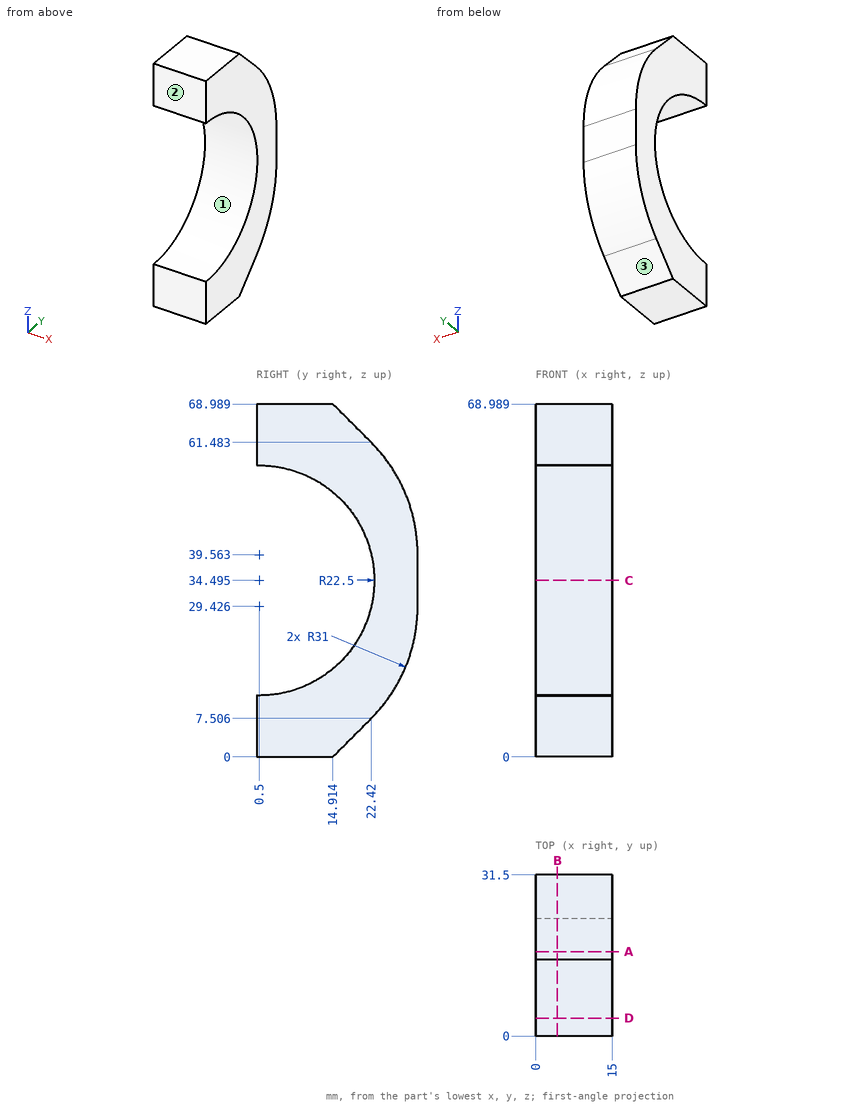
The drawing under review shows one solid part. Ordinate dimensions are in mm from its lowest x, y, z. Round coordinates to 2 decimals unless told otherwise and drop trailing zeros. Loops run counter-clockwise (first coordinate to the right, second up) from the corner with the lowest first, then second, coordinate; pieces in that order, holes last. Notation, with made-up numbers: (-21, 3) - (21, 3) arc R10 cw to (21, 21) - close; hole circle Ø6 at (-26, 18.5). An arc over 180 degrees is marked (long way). Use a Markdown table: item, result. Add a question column.
Q1. Add section B-B (x = 4.25). State the section outline as (y, z) points (1 decimal).
Q2. Add section C-C (z = 34.5). State the section outline as (x, y) points.
Q3. For probe 1 along Z at (x, y) = (9.75, 11) (1 decimal); probe 2 along Z at (x, y) = (6, 8.5) (1 decimal); probe 3 along Y at (x, z) = (14, 28.5) (1 decimal), list the stretches that pass through material, from the lowest coordinate up.
Q4. Add section D-D (y = 3.5). State the section outline as (x, z) points (1 decimal), plus the area to 3 significant figures.
Q5. The part is to be moulded in two halves that separate along Z. For the marked faces 1, 2 and 3, say which applies: pulls with the +Z half, pulls with the -Z half, needs draft (parallel to the pull), parting line crosses it, or undercut.
Q6. Add section A-A (y = 16.5). State the section outline as (x, z) points (1 decimal).
Q7. Insertion check: pin 1 Ø8 at (x, z) = (9, 51.5) entering from +Y; pin 2 Ø6 at (x, z) = (5.5, 16) entering from +Y; pin 3 Ø1 at (x, y) = (2.5, 25.5) entering from -Z. Each pin has a flat end and moves straight along its axis. Give the tip position at first contact, or say it passes through.
Worked answers:
| question | item | result |
|---|---|---|
| 1 | outline | (0, 0) - (14.9, 0) - (22.4, 7.5) arc R31 ccw to (31.5, 29.4) - (31.5, 39.6) arc R31 ccw to (22.4, 61.5) - (14.9, 69) - (0, 69) - (0, 57) arc R22.5 cw (long way) to (0, 12) - close |
| 2 | outline | (0, 23) - (15, 23) - (15, 31.5) - (0, 31.5) - close |
| 3 | probe 1 | 0 to 14.6, 54.4 to 69 |
| 3 | probe 2 | 0 to 13.5, 55.5 to 69 |
| 3 | probe 3 | 22.2 to 31.5 |
| 4 | outline | (0, 0) - (15, 0) - (15, 12.2) - (0, 12.2) - close; (0, 56.8) - (15, 56.8) - (15, 69) - (0, 69) - close |
| 4 | area | 366 mm² |
| 5 | face 1 | undercut |
| 5 | face 2 | needs draft |
| 5 | face 3 | pulls with the -Z half |
| 6 | outline | (0, 1.6) - (15, 1.6) - (15, 18.7) - (0, 18.7) - close; (0, 50.3) - (15, 50.3) - (15, 67.4) - (0, 67.4) - close |
| 7 | pin 1 | y = 30.47 |
| 7 | pin 2 | y = 29.69 |
| 7 | pin 3 | z = 10.43 |
